Autodesk Inventor part; units mm, degrees
ref_plane "Work Plane1" through (3, 0, 0) normal (0, 0, 1) x (1, 0, 0)
ref_plane "YZ Plane" through (0, 0, 0) normal (1, 0, 0) x (0, 1, 0)
ref_plane "XZ Plane" through (0, 0, 0) normal (0, 1, 0) x (-1, 0, 0)
sketch "Sketch1" plane through (0, 0, 0) normal (0, 0, 1) x (1, 0, 0)
  line L0 (0, 0) -> (6, 0)
  line L1 (6, 0) -> (6, 2)
  line L2 (6, 2) -> (0, 2)
  line L3 (0, -0.4) -> (0, 2.4)
  line L4 (0, 2) -> (0, 0)
  dimension "d0" = 4
  dimension "d2" = 6
revolve "Body" add sketch "Sketch1" angle 360 about axis through (0, 0, 0) along (1, 0, 0)
chamfer "Chamfer1" distance 0.4294 angle 45 1 edges at (6, -2, 0) measured on face at (6, 0.2007, 0.5552)
sketch "Sketch2" plane through (0, 0, 0) normal (0, 0, 1) x (1, 0, 0)
  line L0 (6, 1.5706) -> (6, -1.5706)
  line L1 (4.656, 0) -> (6.224, 0)
  line L2 (6, 0.3) -> (4.88, 0.3)
  line L3 (4.88, 0.3) -> (4.88, 0)
  line L4 (4.88, -0.3) -> (4.88, 0)
  line L5 (4.88, -0.3) -> (6, -0.3)
  dimension "d8" = 0.3
  dimension "d9" = 1.12
extrude "Slot1" cut sketch "Sketch2" against normal mid plane 4
thread "Thread"
chamfer "Chamfer2" distance 1.8 angle 45 1 edges at (0, -2, 0) measured on face at (1.8569, -0.8723, 1.7998)
ref_plane "Work Plane1" through (3, 0, 0) normal (0, 0, 1) x (1, 0, 0)
equation "\"d0\" = NND"
equation "\"d2\" = NLG"
equation "\"d8\" = 0.5 * SBR"
equation "\"d9\" = STI"
equation "\"d10\" = NND"
equation "\"d3\" = -0.5 * GD1 + 0.5 * NND"
equation "\"d4\" = FAWI"
equation "\"d34\" = -0.5 * GD1 + 0.5 * NND"
equation "\"d5\" = NLG"
equation "\"d14\" = FAWI"
equation "\"NND\" = 4"
equation "\"NLG\" = 6"
equation "\"FAWI\" = 45deg"
equation "\"GD1\" = THREADDIA - 1.2269 * PTC"
equation "\"FAWI1\" = 45deg"
equation "\"SPD\" = 0.4"
equation "\"SBR\" = 0.6"
equation "\"STI\" = 1.12"
equation "\"GUL\" = 0.61345 * PTC"
equation "\"THREADDIA\" = 4"
equation "\"TOA\" = 30deg"
equation "\"PTC\" = 0.7"
equation "\"GAL\" = 0.61345 * PTC"
equation "\"THREADDESC\" = 1.2345"
properties part number "ISO 7434 - M4x6" material "Stainless Steel, 440C"
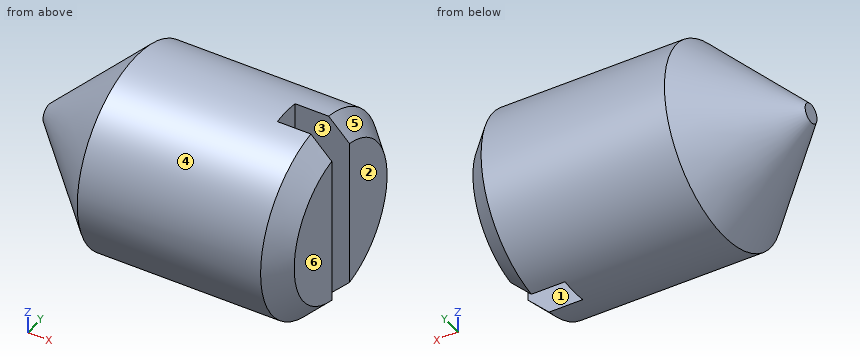
Can you work these out from the model? Positions are in its coordinate system, mm. Face numbers are marked on the shaded views. A direction names the side the tool comes from. Give positions to 0.01 mm unless a question says otherwise; leave off trailing zeros. Order: outer loops, then holes, each group sorted by start corner. A loop starts at its lowest first (then second) coordinate and runs counter-clockwise, first axis right, second up. Notation, with made-up numbers: (-25.75, 16.5) - (12.25, 16.5) arc R6 ccw to (12.25, 23.5) - close; hole circle Ø6 at (38, 33.25). An arc over 180 degrees is marked (long way). Use a Markdown table: item, result. Add a question column.
Q1. If we section it at C-C on y = 0: Write out the boundary of the cut face in (x, z).
Q2. If we section it at D-D on x = 3.5: Write out the boundary of the cut face in (y, z), plus the area to 3 significant figures.
Q3. I'm going to push flat-ended pins straight in: pin 1 (1.5 mm diameter, centred on x = 4, y = -1.5, fed in from -Z); pin 2 (0.6 mm diameter, centred on x = 5.5, z = -0.5, fed in from +Y); pin 3 (1 mm diameter, centred on y = 0, z = 0.5, fed in from +X); pin 4 (0.5 mm diameter, centred on y = 0, z = 1, fed in from +X). Where does each tip first touch, or does it pass through?
Q4. Please list where these lines run through material, in increasing order: line 1 along Z through (x, y) = (2.5, 0.3); line 2 along Y through (x, z) = (5, 1.7); line 3 along Z through (x, y) = (4.25, -0.6).
Q5. If we section it at B-B on x = 5: Write out the boundary of the cut face in (y, z), plus the area to 3 significant figures.
Q6. If we section it at A-A on z = 0: Write out the boundary of the cut face in (x, y).
Q7. If we mould it in two halves opening along Y, with no side actions, what happens to the marked faces 3, 4, 5 and 6? For each: released by +Y, released by -Y, zero draft, split by the parting line, or undercut.
Q8. On a 3-axis mill with a long thin cutter (end or side, diameter ignored), from which of +Z, -Z, +X, -X, +Y, -Y can I reach the whole of each face in a straight line? I mean the marked faces 1 and 2. Say none if no direction works.
Answers follow:
| question | item | result |
|---|---|---|
| 1 | outline | (0, -0.2) - (1.8, -2) - (4.88, -2) - (4.88, 2) - (1.8, 2) - (0, 0.2) - close |
| 2 | outline | circle Ø4 at (0, 0) |
| 2 | area | 12.6 mm^2 |
| 3 | pin 1 | stops at z = -1.85 |
| 3 | pin 2 | stops at y = 1.99 |
| 3 | pin 3 | stops at x = 6 |
| 3 | pin 4 | stops at x = 4.88 |
| 4 | line 1 | z = -1.98 to 1.98 |
| 4 | line 2 | y = -1.05 to -0.3, 0.3 to 1.05 |
| 4 | line 3 | z = -1.91 to 1.91 |
| 5 | outline | (-0.3, -1.98) - (-0.3, 1.98) arc R2 ccw to start; (0.3, -1.98) arc R2 ccw to (0.3, 1.98) - close |
| 5 | area | 10.2 mm^2 |
| 6 | outline | (0, -0.2) - (1.8, -2) - (5.57, -2) - (6, -1.57) - (6, -0.3) - (4.88, -0.3) - (4.88, 0.3) - (6, 0.3) - (6, 1.57) - (5.57, 2) - (1.8, 2) - (0, 0.2) - close |
| 7 | face 3 | undercut |
| 7 | face 4 | split by the parting line |
| 7 | face 5 | released by +Y |
| 7 | face 6 | zero draft |
| 8 | face 1 | +Z, -Z, +X |
| 8 | face 2 | +Z, -Z, +X, +Y, -Y |
